```python
from build123d import *

# Parameters (mm, degrees)
SKETCH5_R           = 7.5
BOSS_EXTRUDE3_DEPTH = 40
SKETCH10_W          = 27.7
SKETCH10_H          = 3.7
CUT_EXTRUDE2_DEPTH  = 15
SKETCH11_W          = 27.7
SKETCH11_H          = 3.7
BOSS_EXTRUDE5_DEPTH = 55


with BuildPart() as part:
    # Sketch5 → Boss-Extrude3 (new body)
    with BuildSketch(Plane.XY):
        Circle(SKETCH5_R)
    extrude(amount=BOSS_EXTRUDE3_DEPTH)

    # Sketch10 → Cut-Extrude2 (cut)
    with BuildSketch(Plane.XY.offset(40)):
        Rectangle(SKETCH10_W, SKETCH10_H)
    extrude(amount=-CUT_EXTRUDE2_DEPTH, mode=Mode.SUBTRACT)

    # Sketch11 → Boss-Extrude5 (add)
    with BuildSketch(Plane.XY.offset(25)):
        Rectangle(SKETCH11_W, SKETCH11_H)
    extrude(amount=BOSS_EXTRUDE5_DEPTH)


solid = part.part
```
Geometry check sheet. Reference: the model listing, model coordinates, mm. A direction names the side the tool comes from. Coordinates: 2 decimals unless noted, no trailing zeros. Loops run counter-clockwise (first coordinate to the right, second up) from the corner with the lowest first, then second, coordinate; pieces in that order, holes last.
Item 1: Sectioned sample at C-C, the plane y = -3.5. Record the boundary of the cut face in (x, z).
Item 2: Go/stop test with flat-tipped pins: pin 1 Ø5 at (x, z) = (-11, 32.5) entering from +Y; pin 2 Ø2 at (x, y) = (-6, -4.5) entering from +Z; pin 3 Ø3 at (x, y) = (11, -1) entering from -Z. Record where each tip stops, or that it passes through.
Item 3: Sectioned sample at A-A, the plane z = 30. Record the boundary of the cut face in (x, y), then the cut area to 3 significant figures.
Item 4: Thickness scan on line 1 (Y direction, x = 0.75, z = 49); line 2 (X direction, y = -0.5, z = 5); line 3 (Z direction, x = -1.5, y = -6). Record the ranges inside material, lowest first.
Item 5: Access from +Z, -Z, +X, -X, +Y, -Y to the whole of each face (thin tool, end or side, straight path). Record for faces 1 (the face through (0, 4, 40)), 2 (the face through (0, -4, 40)), 3 (the face through (0, 0, 0)).
Item 6: Sectioned sample at B-B, the plane x = 0. Record the boundary of the cut face in (y, z), then the cut area to 3 significant figures.
Item 7: Sectioned sample at D-D, the plane x = -8.5. Record the boundary of the cut face in (y, z).
Check result:
1. outline: (-6.63, 0) - (6.63, 0) - (6.63, 40) - (-6.63, 40) - close
2. pin 1: stops at y = 1.85
2. pin 2: stops at z = 40
2. pin 3: stops at z = 25
3. outline: (-13.85, -1.85) - (-7.27, -1.85) arc R7.5 ccw to (7.27, -1.85) - (13.85, -1.85) - (13.85, 1.85) - (7.27, 1.85) arc R7.5 ccw to (-7.27, 1.85) - (-13.85, 1.85) - close
3. area: 224 mm2
4. line 1: y = -1.85 to 1.85
4. line 2: x = -7.48 to 7.48
4. line 3: z = 0 to 40
5. face 1: +Z, +X, -X, +Y
5. face 2: +Z, +X, -X, -Y
5. face 3: -Z, +X, -X, +Y, -Y
6. outline: (-7.5, 0) - (7.5, 0) - (7.5, 40) - (1.85, 40) - (1.85, 80) - (-1.85, 80) - (-1.85, 40) - (-7.5, 40) - close
6. area: 748 mm2
7. outline: (-1.85, 25) - (1.85, 25) - (1.85, 80) - (-1.85, 80) - close
